from build123d import *

# Parameters (mm, degrees)
F2_R      = 62.5
F2_W      = 38.8455463488
F2_H      = 38.8455463488
F3_DEPTH  = 157.39
F8_W      = 38.8455463488
F8_H      = 38.8455463488
F8_W_2    = 35.5
F8_H_2    = 35.5
F9_DEPTH  = 3
F11_DEPTH = 80
F12_R     = 6.35
F13_DEPTH = 12.7


# Not quite as in the source:
# - a feature names something its author has since deleted; it is built from what else it names


with BuildPart() as f1:
    # F0 (on Front) → F1 (revolve)
    with BuildSketch(Plane.XZ):
        with BuildLine():
            ThreePointArc((-62.42, 0), (-60.0517541619, 76.462422463), (-50.8, 152.4))
            Line((-50.8, 152.4), (-45.72, 152.4))
            Line((-45.72, 152.4), (-45.72, 157.4))
            add(Edge.make_bspline(
                [(-75.12, 80), (-74.447497537, 106.2833289956), (-73.373072159, 148.2749606206), (-53.2483071241, 154.9157878093), (-45.72, 157.4)],
                knots=[0, 0, 0, 0, 0.6259182599, 1, 1, 1, 1], degree=3))
            Line((-75.12, 80), (-75.12, 0))
            Line((-75.12, 0), (-62.42, 0))
        make_face()
    revolve(axis=Axis((0, 0, 76.2), (0, 0, 1)))

    # F2 (on Top) → F3 (join)
    with BuildSketch(Plane.XY):
        Circle(F2_R)
        Rectangle(F2_W, F2_H, mode=Mode.SUBTRACT)
    extrude(amount=F3_DEPTH)

    # F5 (on Front) → F6 (revolve, cut)
    with BuildSketch(Plane.XZ):
        with BuildLine():
            Line((-19.432, 0), (0, 0))
            Line((0, 0), (0, 117.132))
            Line((0, 117.132), (-19.432, 117.132))
            add(Edge.make_bspline(
                [(-49.6, 0), (-46.3600523587, 18.5581395922), (-40.1579876774, 54.0830291461), (-27.905682613, 101.3967550255), (-21.7260374714, 112.8720762759), (-19.432, 117.132)],
                knots=[0, 0, 0, 0, 0.4074955134, 0.7800476463, 1, 1, 1, 1], degree=3))
            Line((-49.6, 0), (-19.432, 0))
        make_face()
    revolve(axis=Axis((0, 0, 58.566), (0, 0, -1)), mode=Mode.SUBTRACT)

    # F4 (on Front) → F7 (revolve, cut)
    with BuildSketch(Plane.XZ):
        with BuildLine():
            Line((-59.5792606473, 163.4935438633), (-68.9641386271, 155.4379612207))
            Line((-68.9641386271, 155.4379612207), (-62.5000447035, 148.8302797079))
            ThreePointArc((-62.5000447035, 148.8302797079), (-55.5803045517, 155.0029325492), (-46.5795062482, 157.2322994471))
            Line((-46.5795062482, 157.2322994471), (0, 157.2322994471))
            Line((0, 157.2322994471), (0, 165.5570715666))
            Line((0, 165.5570715666), (-59.5792606473, 163.4935438633))
        make_face()
    revolve(axis=Axis((0, 0, 161.3946855068), (0, 0, 1)), mode=Mode.SUBTRACT)

    # F8 (on face) → F9 (join)
    with BuildSketch(Plane.XY.offset(157.2322994471)):
        Rectangle(F8_W, F8_H)
        Rectangle(F8_W_2, F8_H_2, mode=Mode.SUBTRACT)
    extrude(amount=-F9_DEPTH)

    # F10 (on face) → F11 (cut)
    with BuildSketch(Plane(origin=(0, 0, 0), x_dir=(1, 0, 0), z_dir=(0, 0, -1))):
        with BuildLine():
            Line((-6.35, 62.42), (6.35, 62.42))
            Line((6.35, 62.42), (5.08, 74.9480353312))
            ThreePointArc((5.08, 74.9480353312), (0, 75.12), (-5.08, 74.9480353312))
            Line((-5.08, 74.9480353312), (-6.35, 62.42))
        make_face()
        with BuildLine():
            ThreePointArc((-5.08, 74.9480353312), (0, 75.12), (5.08, 74.9480353312))
            ThreePointArc((5.08, 74.9480353312), (0, 79.5390976959), (-5.08, 74.9480353312))
        make_face()
        with BuildLine():
            Line((-6.35, -62.42), (-5.08, -74.9480353312))
            ThreePointArc((-5.08, -74.9480353312), (0, -75.12), (5.08, -74.9480353312))
            Line((5.08, -74.9480353312), (6.35, -62.42))
            Line((6.35, -62.42), (-6.35, -62.42))
        make_face()
        with BuildLine():
            ThreePointArc((5.08, -74.9480353312), (0, -75.12), (-5.08, -74.9480353312))
            ThreePointArc((-5.08, -74.9480353312), (0, -79.5390976959), (5.08, -74.9480353312))
        make_face()
    extrude(amount=-F11_DEPTH, mode=Mode.SUBTRACT)

    # F12 (on face) → F13 (cut)
    with BuildSketch(Plane(origin=(0, 0, 0), x_dir=(1, 0, 0), z_dir=(0, 0, -1))):
        with Locations((-44.1376052817, 44.1376052817)):
            Circle(F12_R)
        with Locations((44.1376052817, 44.1376052817)):
            Circle(F12_R)
        with Locations((44.1376052817, -44.1376052817)):
            Circle(F12_R)
        with Locations((-44.1376052817, -44.1376052817)):
            Circle(F12_R)
    extrude(amount=-F13_DEPTH, mode=Mode.SUBTRACT)


solid = f1.part
Geometry: final body of the model. Coordinates: model frame, mm. Give positions to 0.01 mm unless a question says otherwise; leave off trailing zeros. Write each question's results on one line, items separated by ' | '.
1) First-contact query: pin 1 Ø2 at (x, y) = (-40, 45.5) entering from +Z; pin 2 Ø4 at (x, y) = (-1.5, 68.5) entering from -Z; pin 3 Ø6.5 at (x, z) = (-1, 31) entering from +Y. Flat tips, straight axial feed; report the tip coordinate or a pass-through.
Geometry says:
pin 1: stops at z = 152.19 | pin 2: stops at z = 80 | pin 3: stops at y = 62.42
2) Cut plane A-A (x = 14). Give the number of separate pieces and of enclosed holes in the cut face, and give its area (3 significant figures).
Geometry says:
separate pieces: 2 | enclosed holes: 2 | area: 12,900 mm²
3) Line query: line 1 along Y through (x, z) = (-18, 37); line 2 along Y through (x, z) = (-2.5, 129.5); line 3 along X through (y, z) = (13, 104.5). Output: solid intervals per line, ascending.
Geometry says:
line 1: y = -72.93 to -38.93, 38.93 to 72.93 | line 2: y = -71.31 to -19.42, 19.42 to 71.31 | line 3: x = -73.1 to -21.96, 21.96 to 73.1
